Check sheet for the modelled part. Datum: model origin and axes. Units: mm. Face numbers are marked on the shaded views. Give positions to 0.01 mm unless a question says otherwise; leave off trailing zeros. Order: outer loops, then holes, each group sorted by start corner. A loop starts at its lowest first (then second) coordinate and runs counter-clockwise, first axis right, second up. Notation, with made-up numbers: (88.5, 65) -> (110.5, 65) arc R21 cw to (110.5, 99) -> close; hole circle Ø10 at (8, 7). An arc over 180 degrees is marked (long way). Write each question's results on one line, items separated by ' | '.
from build123d import *

# Parameters (mm, degrees)
SKETCH1_W                    = 76.2
SKETCH1_H                    = 76.2
BOSS_EXTRUDE1_DEPTH          = 9.525
SKETCH6_R                    = 3.81
CUT_EXTRUDE2_DEPTH           = 2.54
CUT_EXTRUDE2_DRAFT           = 30
CUT_EXTRUDE2_PROFILE_2_DEPTH = 2.54
CUT_EXTRUDE2_PROFILE_2_DRAFT = 30
CUT_EXTRUDE4_REACH           = 56.717
SKETCH12_R                   = 4.064
SKETCH13_R                   = 6.858
CUT_EXTRUDE7_DEPTH           = 3.81
SKETCH7_R                    = 4.445
CUT_EXTRUDE8_DEPTH           = 3.81
CUT_EXTRUDE8_TAPER           = 45
CUT_EXTRUDE9_REACH           = 56.717
SKETCH15_R                   = 4.445
FILLET1_R                    = 2.54
CUT_EXTRUDE10_REACH          = 56.717
SKETCH16_W                   = 29.591
SKETCH16_H                   = 11.1125
SKETCH16_W_2                 = 11.1125
SKETCH16_H_2                 = 29.591
SKETCH17_R                   = 21.59
BOSS_EXTRUDE2_DEPTH          = 9.525
SKETCH18_R                   = 1.3335
BOSS_EXTRUDE3_DEPTH          = 2.54


with BuildPart() as part:
    # Sketch1 → Boss-Extrude1 (new body)
    with BuildSketch(Plane(origin=(0, 0, 0), x_dir=(1, 0, 0), z_dir=(0, 1, 0))):
        Rectangle(SKETCH1_W, SKETCH1_H)
    extrude(amount=BOSS_EXTRUDE1_DEPTH)


with BuildPart() as cut_extrude2_tool:
    # Sketch6 → Cut-Extrude2 (with draft: the straight prism first)
    with BuildSketch(Plane(origin=(0, 0, 0), x_dir=(1, 0, 0), z_dir=(0, 1, 0))):
        with Locations((-28.575, 28.575)):
            Circle(SKETCH6_R)
    extrude(amount=CUT_EXTRUDE2_DEPTH)
    # Cut-Extrude2: the draft: its side faces are tilted about the plane it starts from
    cut_extrude2_sides = [cut_extrude2_tool.faces().sort_by_distance(p)[0] for p in [
        (-32.385, 1.27, -28.575),
    ]]
    draft(cut_extrude2_sides, Plane(origin=(0, 0, 0), x_dir=(1, 0, 0), z_dir=(0, 1, 0)), CUT_EXTRUDE2_DRAFT)


with BuildPart() as part_1:
    add(part.part)

    # Cut-Extrude2: cut by cut_extrude2_tool
    add(cut_extrude2_tool.part, mode=Mode.SUBTRACT)


with BuildPart() as cut_extrude2_profile_2_tool:
    # Sketch6 → Cut-Extrude2 profile 2 (with draft: the straight prism first)
    with BuildSketch(Plane(origin=(0, 0, 0), x_dir=(1, 0, 0), z_dir=(0, 1, 0))):
        with Locations((28.575, -28.575)):
            Circle(SKETCH6_R)
    extrude(amount=CUT_EXTRUDE2_PROFILE_2_DEPTH)
    # Cut-Extrude2 profile 2: the draft: its side faces are tilted about the plane it starts from
    cut_extrude2_profile_2_sides = [cut_extrude2_profile_2_tool.faces().sort_by_distance(p)[0] for p in [
        (24.765, 1.27, 28.575),
    ]]
    draft(cut_extrude2_profile_2_sides, Plane(origin=(0, 0, 0), x_dir=(1, 0, 0), z_dir=(0, 1, 0)), CUT_EXTRUDE2_PROFILE_2_DRAFT)


with BuildPart() as part_2:
    add(part_1.part)

    # Cut-Extrude2 profile 2: cut by cut_extrude2_profile_2_tool
    add(cut_extrude2_profile_2_tool.part, mode=Mode.SUBTRACT)

    # Sketch12 → Cut-Extrude4 (cut, up to next)
    with BuildSketch(Plane(origin=(0, 9.525, 0), x_dir=(1, 0, 0), z_dir=(0, 1, 0)), mode=Mode.PRIVATE) as cut_extrude4_sk1:
        with Locations(Location((-27.94, -6.35, 0), (0, 0, 270))):
            Circle(SKETCH12_R)
    cut_extrude4_tool1 = extrude(cut_extrude4_sk1.sketch, amount=-CUT_EXTRUDE4_REACH, mode=Mode.PRIVATE) & part_2.part
    # Sketch12 → Cut-Extrude4 (cut, up to next)
    with BuildSketch(Plane(origin=(0, 9.525, 0), x_dir=(1, 0, 0), z_dir=(0, 1, 0)), mode=Mode.PRIVATE) as cut_extrude4_sk2:
        with Locations(Location((-6.35, -27.94, 0), (0, 0, 270))):
            Circle(SKETCH12_R)
    cut_extrude4_tool2 = extrude(cut_extrude4_sk2.sketch, amount=-CUT_EXTRUDE4_REACH, mode=Mode.PRIVATE) & part_2.part
    add(cut_extrude4_tool1.solids().sort_by_distance((-27.94, 9.525, 6.35))[0], mode=Mode.SUBTRACT)
    add(cut_extrude4_tool2.solids().sort_by_distance((-6.35, 9.525, 27.94))[0], mode=Mode.SUBTRACT)

    # Sketch13 → Cut-Extrude7 (cut)
    with BuildSketch(Plane.XZ.offset(-9.525)):
        with Locations(Location((-27.94, 6.35, 0), (0, 0, 90))):
            Circle(SKETCH13_R)
        with Locations(Location((-6.35, 27.94, 0), (0, 0, 90))):
            Circle(SKETCH13_R)
    extrude(amount=CUT_EXTRUDE7_DEPTH, mode=Mode.SUBTRACT)

    # Sketch7 → Cut-Extrude8 (cut)
    with BuildSketch(Plane(origin=(0, 0, 0), x_dir=(1, 0, 0), z_dir=(0, 1, 0))):
        with Locations((-27.94, -27.94)):
            Circle(SKETCH7_R)
    extrude(amount=CUT_EXTRUDE8_DEPTH, taper=CUT_EXTRUDE8_TAPER, mode=Mode.SUBTRACT)

    # Sketch15 → Cut-Extrude9 (cut, up to next)
    with BuildSketch(Plane(origin=(0, 9.525, 0), x_dir=(1, 0, 0), z_dir=(0, 1, 0)), mode=Mode.PRIVATE) as cut_extrude9_sk1:
        with Locations(Location((0, 0, 0), (0, 0, 270))):
            Circle(SKETCH15_R)
    cut_extrude9_tool1 = extrude(cut_extrude9_sk1.sketch, amount=-CUT_EXTRUDE9_REACH, mode=Mode.PRIVATE) & part_2.part
    add(cut_extrude9_tool1.solids().sort_by_distance((0, 9.525, 0))[0], mode=Mode.SUBTRACT)

    # Fillet1
    fillet1_edges = [part_2.edges().sort_by_distance(p)[0] for p in [
        (38.1, 4.7625, 38.1),
        (-38.1, 4.7625, 38.1),
        (-38.1, 4.7625, -38.1),
        (38.1, 4.7625, -38.1),
    ]]
    fillet(fillet1_edges, radius=FILLET1_R)

    # Sketch16 → Cut-Extrude10 (cut, up to next)
    with BuildSketch(Plane.XZ, mode=Mode.PRIVATE) as cut_extrude10_sk1:
        with Locations((0, -32.54375)):
            Rectangle(SKETCH16_W, SKETCH16_H)
    cut_extrude10_tool1 = extrude(cut_extrude10_sk1.sketch, amount=-CUT_EXTRUDE10_REACH, mode=Mode.PRIVATE) & part_2.part
    # Sketch16 → Cut-Extrude10 (cut, up to next)
    with BuildSketch(Plane.XZ, mode=Mode.PRIVATE) as cut_extrude10_sk2:
        with Locations((32.54375, 0)):
            Rectangle(SKETCH16_W_2, SKETCH16_H_2)
    cut_extrude10_tool2 = extrude(cut_extrude10_sk2.sketch, amount=-CUT_EXTRUDE10_REACH, mode=Mode.PRIVATE) & part_2.part
    add(cut_extrude10_tool1.solids().sort_by_distance((0, 0, -32.54375))[0], mode=Mode.SUBTRACT)
    add(cut_extrude10_tool2.solids().sort_by_distance((32.54375, 0, 0))[0], mode=Mode.SUBTRACT)

    # Sketch17 → Boss-Extrude2 (add)
    with BuildSketch(Plane(origin=(0, 9.525, 0), x_dir=(1, 0, 0), z_dir=(0, 1, 0))):
        with Locations((36.311274722, 36.311274722)):
            Circle(SKETCH17_R)
    extrude(amount=-BOSS_EXTRUDE2_DEPTH)

    # Sketch18 → Boss-Extrude3 (add)
    with BuildSketch(Plane(origin=(0, 9.525, 0), x_dir=(1, 0, 0), z_dir=(0, 1, 0))):
        with Locations(Location((19.166305808, 41.020673934, 0), (0, 0, 270))):
            Circle(SKETCH18_R)
        with Locations(Location((48.962218533, 48.804553742, 0), (0, 0, 270))):
            Circle(SKETCH18_R)
        with Locations(Location((40.805299824, 19.108596489, 0), (0, 0, 270))):
            Circle(SKETCH18_R)
    extrude(amount=BOSS_EXTRUDE3_DEPTH)


solid = part_2.part
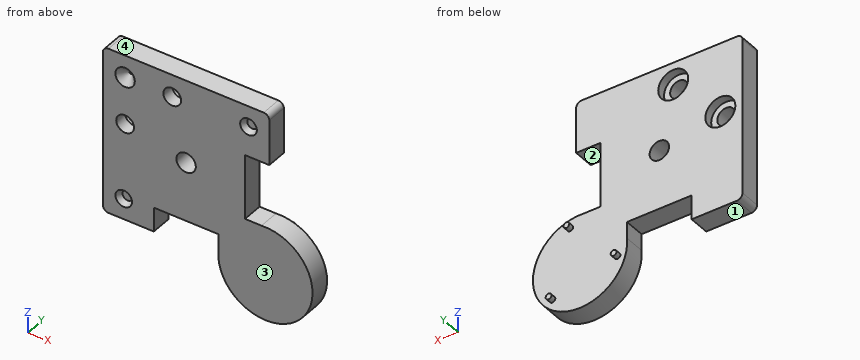
1. Mould release check, pull along Z, two halves, no side actions. Record for the marked faces 1, 2, 3 and 4: +Z half, -Z half, draft (parallel to the pull), parting line (faces both ways), or undercut.
Verdict:
face 1: -Z half | face 2: undercut | face 3: draft | face 4: +Z half
2. Section check C-C on x = 7. Record the cut outline in (y, z) (1 decimal), then the cut area to 3 significant figures.
Verdict:
outline: (0, -27) -> (9.5, -27) -> (9.5, 38.1) -> (0, 38.1) -> close | area: 620 mm^2
3. Section check D-D on y = 10.75. Record the cut outline in (x, z).
Verdict:
outline: circle Ø2.67 at (19.17, -41.02); circle Ø2.67 at (40.81, -19.11); circle Ø2.67 at (48.96, -48.8)
4. Gauge pin test, flat ends, axial feed: pin 1 Ø10.5 at (x, z) = (-6.35, 27.94) entering from +Y (3 decimals); pin 2 Ø12 at (x, z) = (13.5, -7.5) entering from +Y (3 decimals); pin 3 Ø1.4 at (x, z) = (-28, 28) entering from -Y. Record the tip position at first contact, or that the pin passes through.
Verdict:
pin 1: stops at y = 5.715 | pin 2: stops at y = 9.525 | pin 3: stops at y = 3.66
5. Material ranges on probe 1 along Z at (x, y) = (-27.94, 8.4); probe 2 along X at (y, z) = (3.2, 27.94) (3 decimals); probe 3 along Z at (x, y) = (-1, 2), recorded low to high. Write a range as from..to.
Verdict:
probe 1: z = -38.1..-0.51, 13.21..38.1 | probe 2: x = -38.1..-29.185, -26.695..-10.414, -2.286..38.1 | probe 3: z = -26.99..-4.33, 4.33..38.1
6. Section check B-B on z = 6.35. Record the cut outline in (x, y) (1 decimal).
Verdict:
outline: (-38.1, 0) -> (-32, 0) -> (-32, 5.7) -> (-34.8, 5.7) -> (-34.8, 9.5) -> (-38.1, 9.5) -> close; (-23.9, 0) -> (27, 0) -> (27, 9.5) -> (-21.1, 9.5) -> (-21.1, 5.7) -> (-23.9, 5.7) -> close
7. Section check A-A on x = -6.35. Record the cut outline in (y, z) (1 decimal), then the cut area to 3 significant figures.
Verdict:
outline: (0, -27) -> (9.5, -27) -> (9.5, 21.1) -> (5.7, 21.1) -> (5.7, 23.9) -> (0, 23.9) -> close; (0, 32) -> (5.7, 32) -> (5.7, 34.8) -> (9.5, 34.8) -> (9.5, 38.1) -> (0, 38.1) -> close | area: 521 mm^2
